Source: CAD feature listing. Evaluate the final solid. Frame: model axes, mm. Face numbers are marked on the shaded views. A direction names the side the tool comes from. Coordinates: 2 decimals unless noted, no trailing zeros. Order: outer loops, then holes, each group sorted by start corner. A loop starts at its lowest first (then second) coordinate and runs counter-clockwise, first axis right, second up. Notation, with made-up numbers: (51, -36) - (76, -36) arc R31 cw to (76, -3) - close; hole circle Ø10 at (24, 55). An arc over 180 degrees is marked (long way). One line per question, with ' | ' between items. Start each with the question number.
(1) Section C-C (x = 3). Return the cut outline in (y, z).
(2) Section A-A (x = 11). Return the cut outline in (y, z), then the cut area to 3 significant figures.
(3) Line query: line 1 along Y through (x, z) = (0, -12.5); line 2 along Y through (x, z) = (-18, 33); line 3 along X through (y, z) = (10, -18.5). Output: solid intervals per line, ascending.
(4) Section D-D (y = -27.5). Return the cut outline in (x, z), then the cut area to 3 significant figures.
(5) Section B-B (z = -13). Return the cut outline in (x, y), then the cut area to 3 significant figures.
(6) Draft query along X for the marked faces 4, 5, 6 and 7. Return one class per face: +X half, -X half, draft (parallel to the pull), parting line (faces both ways), or undercut.
(7) Contact query for flat-ended pins moving along their axis: P1, Ø11.5, axis at x = 0.5, y = -6.5, coming from the +Z side; P2, Ø3, axis at x = 13.5, z = 24.5, coming from the +Y side; P3, Ø3, axis at x = -8.5, y = 4, coming from the -Z side. Output: stop coordinate, or through.
(8) Access query for the marked faces 1, 2 and 3. Directions: +Z, -Z, +X, -X, +Y, -Y. A direction counts if a zero-diameter tool reaches every point of the face in a straight line with its end or side. Return the directions, or none.
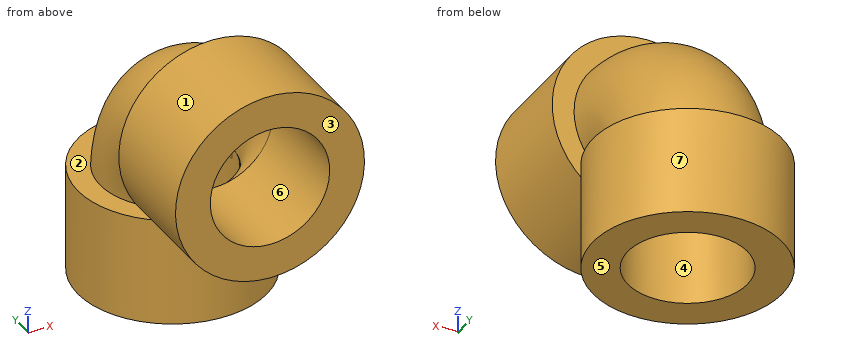
from build123d import *

# Parameters (mm, degrees)
ESQUISSE1_R             = 16.9
ESQUISSE1_R_2           = 13.9
R_VOL_MINCE1_ANGLE      = 90
ESQUISSE2_R             = 15.9
ESQUISSE2_R_2           = 13.9
EXTRU_MINCE1_DEPTH      = 22.4
ESQUISSE3_R             = 18.1
ESQUISSE3_R_2           = 16.1
EXTRU_MINCE2_DEPTH      = 22.3
CROQUIS1_R              = 22
CROQUIS1_R_2            = 13.9
SALIENTE_EXTRUIR1_DEPTH = 25
SALIENTE_EXTRUIR2_START = -25
CROQUIS2_R              = 22
CROQUIS2_R_2            = 13.9
SALIENTE_EXTRUIR2_DEPTH = 25


with BuildPart() as part:
    # Esquisse1 → Révol.-Mince1 (revolve)
    with BuildSketch(Plane.XY):
        Circle(ESQUISSE1_R)
        Circle(ESQUISSE1_R_2, mode=Mode.SUBTRACT)
    revolve(axis=Axis((0, -20.745281933, 0), (1, 0, 0)), revolution_arc=R_VOL_MINCE1_ANGLE)

    # Esquisse2 → Extru.-Mince1 (add)
    with BuildSketch(Plane(origin=(0, 0, 0), x_dir=(-1, 0, 0), z_dir=(0, 0, -1))):
        Circle(ESQUISSE2_R)
        Circle(ESQUISSE2_R_2, mode=Mode.SUBTRACT)
    extrude(amount=EXTRU_MINCE1_DEPTH)

    # Esquisse3 → Extru.-Mince2 (add)
    with BuildSketch(Plane.XZ.offset(20.745281933)):
        with Locations((0, 20.745281933)):
            Circle(ESQUISSE3_R)
        with Locations((0, 20.745281933)):
            Circle(ESQUISSE3_R_2, mode=Mode.SUBTRACT)
    extrude(amount=EXTRU_MINCE2_DEPTH)

    # Croquis1 → Saliente-Extruir1 (add)
    with BuildSketch(Plane.XZ.offset(43.045281933)):
        with Locations(Location((0, 20.745281933, 0), (0, 0, 270))):
            Circle(CROQUIS1_R)
        with Locations(Location((0, 20.745281933, 0), (0, 0, 270))):
            Circle(CROQUIS1_R_2, mode=Mode.SUBTRACT)
    extrude(amount=-SALIENTE_EXTRUIR1_DEPTH)

    # Croquis2 → Saliente-Extruir2 (add)
    with BuildSketch(Plane(origin=(0, 0, -22.4), x_dir=(-1, 0, 0), z_dir=(0, 0, -1)).offset(SALIENTE_EXTRUIR2_START)):
        Circle(CROQUIS2_R)
        Circle(CROQUIS2_R_2, mode=Mode.SUBTRACT)
    extrude(amount=SALIENTE_EXTRUIR2_DEPTH)


solid = part.part
Response values:
1) outline: (-43.05, -1.05) - (-21.79, -1.05) - (-21.79, -22.4) - (-13.57, -22.4) - (-13.57, 2.6) - (-14.06, 2.6) arc R7.17 ccw to (-18.05, 6.65) - (-18.05, 7.17) - (-43.05, 7.17) - close; (-43.05, 34.32) - (-20.75, 34.32) arc R34.32 cw to (13.57, 0) - (13.57, -22.4) - (21.79, -22.4) - (21.79, 2.6) - (16.54, 2.6) arc R37.38 ccw to (-18.05, 37.28) - (-18.05, 42.54) - (-43.05, 42.54) - close; hole (-18.05, 2.6) - (-17.56, 2.6) arc R4.11 ccw to (-18.05, 3.1) - close
2) outline: (-43.05, 1.69) - (-19.05, 1.69) - (-19.05, -22.4) - (-8.5, -22.4) - (-8.5, 2.6) - (-8.78, 2.6) arc R12.25 ccw to (-18.05, 11.95) - (-18.05, 12.25) - (-43.05, 12.25) - close; (-43.05, 29.24) - (-20.75, 29.24) arc R29.24 cw to (8.5, 0) - (8.5, -22.4) - (19.05, -22.4) - (19.05, 2.6) - (12.73, 2.6) arc R33.58 ccw to (-18.05, 33.47) - (-18.05, 39.8) - (-43.05, 39.8) - close; hole (-18.05, 2.6) - (-13.27, 2.6) arc R7.92 ccw to (-18.05, 7.44) - close | area: 1,290 mm²
3) line 1: y = -22 to -13.9, 13.9 to 22 | line 2: y = -43.05 to -18.05 | line 3: x = -19.6 to -9.65, 9.65 to 19.6
4) outline: circle Ø44 at (0, 20.75); hole circle Ø27.8 at (0, 20.75) | area: 914 mm²
5) outline: circle Ø44 at (0, 0); hole circle Ø27.8 at (0, 0) | area: 914 mm²
6) face 4: undercut | face 5: draft | face 6: undercut | face 7: parting line
7) P1: stops at z = 36.67 | P2: stops at y = 1.36 | P3: stops at z = 16.87
8) face 1: -Y | face 2: none | face 3: +Z, -Z, +X, -X, -Y
